Part model, mm, in its own coordinate system. Coordinates: 2 decimals unless noted, no trailing zeros. Order: outer loops, then holes, each group sorted by start corner. A loop starts at its lowest first (then second) coordinate and runs counter-clockwise, first axis right, second up.
from build123d import *

# Parameters (mm, degrees)
CROQUIS1_R              = 1.25
SALIENTE_EXTRUIR1_DEPTH = 3
CHAFL_N1_SIZE           = 0.5


with BuildPart() as part:
    # Croquis1 → Saliente-Extruir1 (new body)
    with BuildSketch(Plane.XY):
        with BuildLine():
            Line((0, 3), (30, 3))
            ThreePointArc((30, 3), (33, 0), (30, -3))
            Line((30, -3), (0, -3))
            ThreePointArc((0, -3), (-3, 0), (0, 3))
        make_face()
        with Locations((30, 0)):
            Circle(CROQUIS1_R, mode=Mode.SUBTRACT)
        Circle(CROQUIS1_R, mode=Mode.SUBTRACT)
    extrude(amount=SALIENTE_EXTRUIR1_DEPTH)

    # Chaflán1
    chafl_n1_edges = [part.edges().sort_by_distance(p)[0] for p in [
        (33, 0, 3),
        (15, 3, 3),
        (-3, 0, 3),
        (15, -3, 3),
    ]]
    chamfer(chafl_n1_edges, length=CHAFL_N1_SIZE)


solid = part.part
Q1. Pin check, flat tip, straight feed: pin 1 Ø3 at (x, y) = (20.5, 1.5) entering from -Z. Stop position of the tip, or through.
Results list:
pin 1: stops at z = 0
Q2. Cut at A-A on y = 0. Write the cut outline in (x, z), and give its area (4 significant figures).
Results list:
outline: (-3, 0) - (-1.25, 0) - (-1.25, 3) - (-2.5, 3) - (-3, 2.5) - close; (1.25, 0) - (28.75, 0) - (28.75, 3) - (1.25, 3) - close; (31.25, 0) - (33, 0) - (33, 2.5) - (32.5, 3) - (31.25, 3) - close
area: 92.75 mm2
Q3. Cut at B-B on z = 1.4. Write the cut outline in (x, y), and give its area (3 significant figures).
Results list:
outline: (0, -3) - (30, -3) arc R3 ccw to (30, 3) - (0, 3) arc R3 ccw to start; hole circle Ø2.5 at (0, 0); hole circle Ø2.5 at (30, 0)
area: 198 mm2
Q4. Wall check: line 1 along X through (y, z) = (-0.45, 1.7); line 2 along Y through (x, z) = (30, 1.35); line 3 along X through (y, z) = (0.75, 1.3). Give the ranges that are in metal, low to high.
Results list:
line 1: x = -2.97 to -1.17, 1.17 to 28.83, 31.17 to 32.97
line 2: y = -3 to -1.25, 1.25 to 3
line 3: x = -2.9 to -1, 1 to 29, 31 to 32.9
Q5. Mould opens along X. For faces 1 (the face through (33, 0, 1)), 2 (the face through (15, 0, 3)), 3 (the face through (31.155, -0.479, 1.479)) say: pulls with the +X half, pulls with the -X half, needs draft (parallel to the pull), parting line crosses it, or undercut.
Results list:
face 1: pulls with the +X half
face 2: needs draft
face 3: undercut
